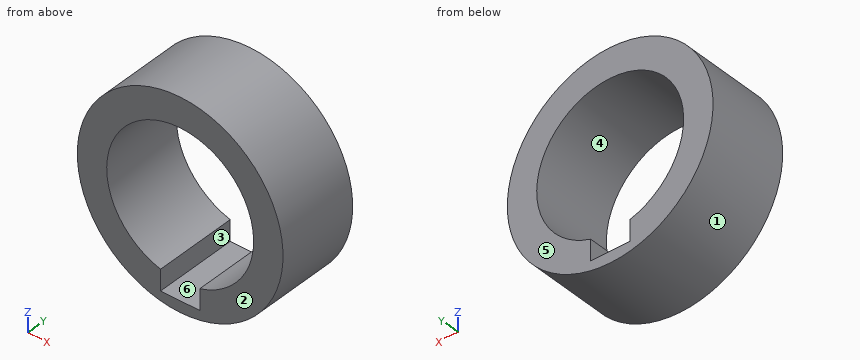
```python
from build123d import *

# Parameters (mm, degrees)
SKETCH1_R           = 21
SKETCH1_R_2         = 15
BOSS_EXTRUDE1_DEPTH = 17
CUT_EXTRUDE1_DEPTH  = 35.219877265


with BuildPart() as part:
    # Sketch1 → Boss-Extrude1 (new body)
    with BuildSketch(Plane(origin=(0, 0, 0), x_dir=(1, 0, 0), z_dir=(0, 1, 0))):
        with Locations(Location((0, 0, 0), (0, 0, 270))):
            Circle(SKETCH1_R)
        with Locations(Location((0, 0, 0), (0, 0, 270))):
            Circle(SKETCH1_R_2, mode=Mode.SUBTRACT)
    extrude(amount=-BOSS_EXTRUDE1_DEPTH)

    # Sketch2 → Cut-Extrude1 (cut, through all)
    with BuildSketch(Plane(origin=(0, 0, 0), x_dir=(1, 0, 0), z_dir=(0, 1, 0))):
        with BuildLine():
            Line((4, 18.7), (-4, 18.7))
            Line((-4, 18.7), (-4, 14.456832295))
            ThreePointArc((-4, 14.456832295), (0, 15), (4, 14.456832295))
            Line((4, 14.456832295), (4, 18.7))
        make_face()
    extrude(amount=-CUT_EXTRUDE1_DEPTH, mode=Mode.SUBTRACT)


solid = part.part
```
Could you check a few things on this model? Use its own coordinates, in mm. Face numbers are marked on the shaded views. A direction names the side the tool comes from. Round coordinates to 2 decimals unless told otherwise and drop trailing zeros. Loops run counter-clockwise (first coordinate to the right, second up) from the corner with the lowest first, then second, coordinate; pieces in that order, holes last.
Q1. Thinking about a two-plate mould opening in Z: for the marked faces 1, 2, 3 and 4, which applies, pulls with the +Z half, pulls with the -Z half, needs draft (parallel to the pull), parting line crosses it, or undercut?
Q2. I want a section at D-D (z = 16). Write out the boundary of the cut face in (x, y), and give its area (3 significant figures).
Q3. I want a section at B-B (z = 0). Write out the boundary of the cut face in (x, y), and give its area (3 significant figures).
Q4. For P1, Ø1, axis at x = -13.5, y = -14.5, coming from the -Z side; P2, Ø2.5, axis at x = -1.5, y = -7, coming from the +Z side; P3, Ø6, axis at x = -8, y = -3.5, coming from the -Z side, each with a flat end and sliding along its axis, tell me the tip position at first contact or that it passes through.
Q5. I want a section at A-A (y = -6.5). Write out the boundary of the cut face in (x, z).
Q6. Please list where these lines run through material, in increasing order: L1, parallel to X at y = -5.5, z = 0; L2, parallel to X at y = -2.75, z = 11; L3, parallel to Z at x = -13.5, y = -2.
Q7. On a 3-axis mill with a long thin cutter (end or side, diameter ignored), from which of +Z, -Z, +X, -X, +Y, -Y can I reach the whole of each face in a straight line? I mean the marked faces 5 and 6. Say none if no direction works.
Q8. I want a section at C-C (x = -5). Write out the boundary of the cut face in (y, z), and give its area (3 significant figures).
Answer below:
1. face 1: parting line crosses it
1. face 2: needs draft
1. face 3: undercut
1. face 4: undercut
2. outline: (-13.6, -17) - (13.6, -17) - (13.6, 0) - (-13.6, 0) - close
2. area: 462 mm2
3. outline: (-21, -17) - (-15, -17) - (-15, 0) - (-21, 0) - close; (15, -17) - (21, -17) - (21, 0) - (15, 0) - close
3. area: 204 mm2
4. P1: stops at z = -16.49
4. P2: stops at z = 21
4. P3: stops at z = -20.4
5. outline: circle Ø42 at (0, 0); hole (-4, -18.7) - (4, -18.7) - (4, -14.46) arc R15 ccw (long way) to (-4, -14.46) - close
6. L1: x = -21 to -15, 15 to 21
6. L2: x = -17.89 to -10.2, 10.2 to 17.89
6. L3: z = -16.09 to -6.54, 6.54 to 16.09
7. face 5: +Z, -Z, +X, -X, +Y
7. face 6: +Y, -Y
8. outline: (-17, -20.4) - (0, -20.4) - (0, -14.14) - (-17, -14.14) - close; (-17, 14.14) - (0, 14.14) - (0, 20.4) - (-17, 20.4) - close
8. area: 213 mm2
